Check sheet for the modelled part. Datum: model origin and axes. Units: mm. Give positions to 0.01 mm unless a question says otherwise; leave off trailing zeros. Order: outer loops, then holes, each group sorted by start corner. A loop starts at its lowest first (then second) coordinate and runs counter-clockwise, first axis right, second up.
```python
from build123d import *

# Parameters (mm, degrees)
SKETCH1_R           = 7.5
BOSS_EXTRUDE1_DEPTH = 0.2


with BuildPart() as part:
    # Sketch1 → Boss-Extrude1 (new body)
    with BuildSketch(Plane(origin=(0, 0, 0), x_dir=(1, 0, 0), z_dir=(0, 1, 0))):
        with Locations(Location((0, 0, 0), (0, 0, 270))):
            Circle(SKETCH1_R)
        with BuildLine():
            Line((4.270625279, -0.564175126), (5.348769596, -1.010757124))
            ThreePointArc((5.348769596, -1.010757124), (5.568208781, -0.997000043), (5.69191502, -0.815232116))
            ThreePointArc((5.69191502, -0.815232116), (5.735460372, -0.408649381), (5.75, 0))
            ThreePointArc((5.75, 0), (5.735460372, 0.408649381), (5.69191502, 0.815232116))
            ThreePointArc((5.69191502, 0.815232116), (5.568208781, 0.997000043), (5.348769596, 1.010757124))
            Line((5.348769596, 1.010757124), (4.270625279, 0.564175126))
            ThreePointArc((4.270625279, 0.564175126), (4.05620803, 0.575146612), (3.929368867, 0.748371773))
            ThreePointArc((3.929368867, 0.748371773), (3.832459783, 1.145535689), (3.69551813, 1.530733729))
            ThreePointArc((3.69551813, 1.530733729), (3.519974355, 1.899942247), (3.307662127, 2.249304616))
            ThreePointArc((3.307662127, 2.249304616), (3.274862273, 2.461482135), (3.418720152, 2.620856037))
            Line((3.418720152, 2.620856037), (4.496864469, 3.067438036))
            ThreePointArc((4.496864469, 3.067438036), (4.642303679, 3.232332697), (4.601247866, 3.448335552))
            ThreePointArc((4.601247866, 3.448335552), (4.344541671, 3.766624174), (4.065863992, 4.065863992))
            ThreePointArc((4.065863992, 4.065863992), (3.766624174, 4.344541671), (3.448335552, 4.601247866))
            ThreePointArc((3.448335552, 4.601247866), (3.232332697, 4.642303679), (3.067438036, 4.496864469))
            Line((3.067438036, 4.496864469), (2.620856037, 3.418720152))
            ThreePointArc((2.620856037, 3.418720152), (2.461482135, 3.274862273), (2.249304616, 3.307662127))
            ThreePointArc((2.249304616, 3.307662127), (1.899942247, 3.519974355), (1.530733729, 3.69551813))
            ThreePointArc((1.530733729, 3.69551813), (1.145535689, 3.832459783), (0.748371773, 3.929368867))
            ThreePointArc((0.748371773, 3.929368867), (0.575146612, 4.05620803), (0.564175126, 4.270625279))
            Line((0.564175126, 4.270625279), (1.010757124, 5.348769596))
            ThreePointArc((1.010757124, 5.348769596), (0.997000043, 5.568208781), (0.815232116, 5.69191502))
            ThreePointArc((0.815232116, 5.69191502), (0.408649381, 5.735460372), (0, 5.75))
            ThreePointArc((0, 5.75), (-0.408649381, 5.735460372), (-0.815232116, 5.69191502))
            ThreePointArc((-0.815232116, 5.69191502), (-0.997000043, 5.568208781), (-1.010757124, 5.348769596))
            Line((-1.010757124, 5.348769596), (-0.564175126, 4.270625279))
            ThreePointArc((-0.564175126, 4.270625279), (-0.575146612, 4.05620803), (-0.748371773, 3.929368867))
            ThreePointArc((-0.748371773, 3.929368867), (-1.145535689, 3.832459783), (-1.530733729, 3.69551813))
            ThreePointArc((-1.530733729, 3.69551813), (-1.899942247, 3.519974355), (-2.249304616, 3.307662127))
            ThreePointArc((-2.249304616, 3.307662127), (-2.461482135, 3.274862273), (-2.620856037, 3.418720152))
            Line((-2.620856037, 3.418720152), (-3.067438036, 4.496864469))
            ThreePointArc((-3.067438036, 4.496864469), (-3.232332697, 4.642303679), (-3.448335552, 4.601247866))
            ThreePointArc((-3.448335552, 4.601247866), (-3.766624174, 4.344541671), (-4.065863992, 4.065863992))
            ThreePointArc((-4.065863992, 4.065863992), (-4.344541671, 3.766624174), (-4.601247866, 3.448335552))
            ThreePointArc((-4.601247866, 3.448335552), (-4.642303679, 3.232332697), (-4.496864469, 3.067438036))
            Line((-4.496864469, 3.067438036), (-3.418720152, 2.620856037))
            ThreePointArc((-3.418720152, 2.620856037), (-3.274862273, 2.461482135), (-3.307662127, 2.249304616))
            ThreePointArc((-3.307662127, 2.249304616), (-3.519974355, 1.899942247), (-3.69551813, 1.530733729))
            ThreePointArc((-3.69551813, 1.530733729), (-3.832459783, 1.145535689), (-3.929368867, 0.748371773))
            ThreePointArc((-3.929368867, 0.748371773), (-4.05620803, 0.575146612), (-4.270625279, 0.564175126))
            Line((-4.270625279, 0.564175126), (-5.348769596, 1.010757124))
            ThreePointArc((-5.348769596, 1.010757124), (-5.568208781, 0.997000043), (-5.69191502, 0.815232116))
            ThreePointArc((-5.69191502, 0.815232116), (-5.735460372, 0.408649381), (-5.75, 0))
            ThreePointArc((-5.75, 0), (-5.735460372, -0.408649381), (-5.69191502, -0.815232116))
            ThreePointArc((-5.69191502, -0.815232116), (-5.568208781, -0.997000043), (-5.348769596, -1.010757124))
            Line((-5.348769596, -1.010757124), (-4.270625279, -0.564175126))
            ThreePointArc((-4.270625279, -0.564175126), (-4.05620803, -0.575146612), (-3.929368867, -0.748371773))
            ThreePointArc((-3.929368867, -0.748371773), (-3.832459783, -1.145535689), (-3.69551813, -1.530733729))
            ThreePointArc((-3.69551813, -1.530733729), (-3.519974355, -1.899942247), (-3.307662127, -2.249304616))
            ThreePointArc((-3.307662127, -2.249304616), (-3.274862273, -2.461482135), (-3.418720152, -2.620856037))
            Line((-3.418720152, -2.620856037), (-4.496864469, -3.067438036))
            ThreePointArc((-4.496864469, -3.067438036), (-4.642303679, -3.232332697), (-4.601247866, -3.448335552))
            ThreePointArc((-4.601247866, -3.448335552), (-4.344541671, -3.766624174), (-4.065863992, -4.065863992))
            ThreePointArc((-4.065863992, -4.065863992), (-3.766624174, -4.344541671), (-3.448335552, -4.601247866))
            ThreePointArc((-3.448335552, -4.601247866), (-3.232332697, -4.642303679), (-3.067438036, -4.496864469))
            Line((-3.067438036, -4.496864469), (-2.620856037, -3.418720152))
            ThreePointArc((-2.620856037, -3.418720152), (-2.461482135, -3.274862273), (-2.249304616, -3.307662127))
            ThreePointArc((-2.249304616, -3.307662127), (-1.899942247, -3.519974355), (-1.530733729, -3.69551813))
            ThreePointArc((-1.530733729, -3.69551813), (-1.145535689, -3.832459783), (-0.748371773, -3.929368867))
            ThreePointArc((-0.748371773, -3.929368867), (-0.575146612, -4.05620803), (-0.564175126, -4.270625279))
            Line((-0.564175126, -4.270625279), (-1.010757124, -5.348769596))
            ThreePointArc((-1.010757124, -5.348769596), (-0.997000043, -5.568208781), (-0.815232116, -5.69191502))
            ThreePointArc((-0.815232116, -5.69191502), (-0.408649381, -5.735460372), (0, -5.75))
            ThreePointArc((0, -5.75), (0.408649381, -5.735460372), (0.815232116, -5.69191502))
            ThreePointArc((0.815232116, -5.69191502), (0.997000043, -5.568208781), (1.010757124, -5.348769596))
            Line((1.010757124, -5.348769596), (0.564175126, -4.270625279))
            ThreePointArc((0.564175126, -4.270625279), (0.575146612, -4.05620803), (0.748371773, -3.929368867))
            ThreePointArc((0.748371773, -3.929368867), (1.145535689, -3.832459783), (1.530733729, -3.69551813))
            ThreePointArc((1.530733729, -3.69551813), (1.899942247, -3.519974355), (2.249304616, -3.307662127))
            ThreePointArc((2.249304616, -3.307662127), (2.461482135, -3.274862273), (2.620856037, -3.418720152))
            Line((2.620856037, -3.418720152), (3.067438036, -4.496864469))
            ThreePointArc((3.067438036, -4.496864469), (3.232332697, -4.642303679), (3.448335552, -4.601247866))
            ThreePointArc((3.448335552, -4.601247866), (3.766624174, -4.344541671), (4.065863992, -4.065863992))
            ThreePointArc((4.065863992, -4.065863992), (4.344541671, -3.766624174), (4.601247866, -3.448335552))
            ThreePointArc((4.601247866, -3.448335552), (4.642303679, -3.232332697), (4.496864469, -3.067438036))
            Line((4.496864469, -3.067438036), (3.418720152, -2.620856037))
            ThreePointArc((3.418720152, -2.620856037), (3.274862273, -2.461482135), (3.307662127, -2.249304616))
            ThreePointArc((3.307662127, -2.249304616), (3.519974355, -1.899942247), (3.69551813, -1.530733729))
            ThreePointArc((3.69551813, -1.530733729), (3.832459783, -1.145535689), (3.929368867, -0.748371773))
            ThreePointArc((3.929368867, -0.748371773), (4.05620803, -0.575146612), (4.270625279, -0.564175126))
        make_face(mode=Mode.SUBTRACT)
    extrude(amount=BOSS_EXTRUDE1_DEPTH)


solid = part.part
```
(1) Cross-section at B-B on z = 1.25. Enter the section's corners in (x, y).
Response values:
outline: (-7.4, 0) - (-3.8, 0) - (-3.8, 0.2) - (-7.4, 0.2) - close; (3.8, 0) - (7.4, 0) - (7.4, 0.2) - (3.8, 0.2) - close
(2) Material ranges on L1, parallel to Z at x = -4.5, y = 0.1; L2, parallel to X at y = 0.15, z = 4.25; L3, parallel to Z at x = 6, y = 0.1, recorded low to high.
Response values:
L1: z = -6 to -3.58, -3.07 to -0.66, 0.66 to 3.07, 3.58 to 6
L2: x = -6.18 to -3.87, -2.97 to -0.56, 0.56 to 2.97, 3.87 to 6.18
L3: z = -4.5 to 4.5
(3) Cross-section at A-A on x = 1.25. Enter the section's corners in (y, z).
Response values:
outline: (0, -7.4) - (0.2, -7.4) - (0.2, -3.8) - (0, -3.8) - close; (0, 3.8) - (0.2, 3.8) - (0.2, 7.4) - (0, 7.4) - close
